Autodesk Inventor part; units mm, degrees
ref_plane "YZ Plane" through (0, 0, 0) normal (1, 0, 0) x (0, 1, 0)
ref_plane "XZ Plane" through (0, 0, 0) normal (0, 1, 0) x (-1, 0, 0)
ref_plane "XY Plane" through (0, 0, 0) normal (0, 0, 1) x (1, 0, 0)
sketch "Sketch1" plane through (0, 0, 0) normal (0, 0, 1) x (1, 0, 0)
  line L0 (-85, 50) -> (85, 50)
  line L1 (85, 50) -> (85, -50)
  line L2 (85, -50) -> (-85, -50)
  line L3 (-85, -50) -> (-85, 50)
  line L4 (-85, 50) -> (85, -50) construction
  line L5 (85, 50) -> (-85, -50) construction
  point P0 (0, 0)
  dimension "d0" = 170
  dimension "d1" = 100
extrude "Extrusion1" add sketch "Sketch1" along normal mid plane 10
sketch "Sketch2" plane through (0, 0, 5) normal (0, 0, 1) x (1, 0, 0)
  line L0 (-85, 50) -> (-85, -50)
  line L1 (-85, -50) -> (85, -50)
  line L2 (85, -50) -> (85, 50)
  line L3 (85, 50) -> (-85, 50)
  point P0 (0, 0)
  point P1 (-80, -45)
  point P2 (0, -45)
  point P3 (-55, -45)
  point P4 (55, -45)
  point P5 (0, -45)
  point P6 (80, -45)
  point P7 (-80, 0)
  point P8 (80, 0)
  point P9 (-80, 45)
  point P10 (80, 45)
  point P11 (-55, 45)
  point P12 (0, 45)
  point P13 (55, 45)
  dimension "d4" = 5
  dimension "d5" = 5
  dimension "d8" = 80
  dimension "d13" = 25
  dimension "d14" = 5
  dimension "d16" = 5
  dimension "d60" = 5
  dimension "d61" = 5
  dimension "d62" = 25
  dimension "d65" = 45
  dimension "d72" = 90
hole "Hole1" at (-80, -45, 5) at (0, -45, 5) at (-55, -45, 5) at (55, -45, 5) at (-80, 45, 5) at (-80, 0, 5) at (-55, 45, 5) at (0, 45, 5) at (55, 45, 5) at (80, 45, 5) at (80, 0, 5) at (80, -45, 5) direction (0, 0, -1) diameter 3.242 end through all
sketch "Sketch3" plane through (0, 0, 5) normal (0, 0, 1) x (1, 0, 0)
  point P0 (0, 0)
  point P1 (0, 15)
  point P2 (-15, 0)
  point P3 (0, -15)
  point P4 (15, 0)
  dimension "d105" = 15
  dimension "d108" = 360
hole "Hole2" at (0, 15, 5) at (-15, 0, 5) at (0, -15, 5) at (15, 0, 5) direction (0, 0, -1) diameter 3 depth 5 tip angle 118
properties part number "topwindow"
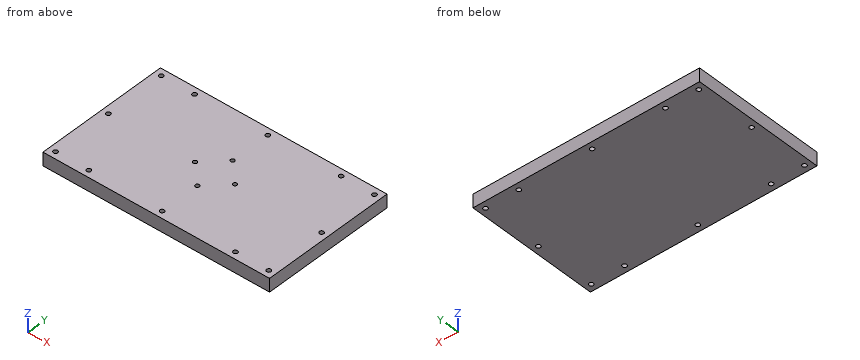
Geometry check sheet. Reference: the model listing, model coordinates, mm. Round coordinates to 2 decimals unless told otherwise and drop trailing zeros. Write each loop counter-clockwise with the first axis right and the second up, starting at its lowest first coordinate (ties: lowest second). Pieces come first, ordered by that corner, then holes. Notation, with made-up numbers: (43, 21) -> (61, 21) arc R13 cw to (61, 39) -> close; hole circle Ø4 at (13, 7.25). An arc over 180 degrees is marked (long way). One line per item, written item: value. Start each with the question number.
(1) Scan lines: line 1 (Y direction, x = 0, z = 2.9); line 2 (X direction, y = 45, z = 0.5); line 3 (X direction, y = 0, z = 3.55). Record each from-to range of solid material in increasing order. Write a range as [from, to].
(2) Cross-section at A-A, the plane x = 80. Record the cut outline in (y, z), and give its area (3 significant figures).
(3) Cross-section at B-B, the plane x = 55. Record the cut outline in (y, z), and give its area (3 significant figures).
(4) Go/stop test with flat-tipped pins: pin 1 Ø1.8 at (x, y) = (0, 15) entering from +Z; pin 2 Ø2.5 at (x, y) = (-15, 0) entering from +Z. Record where each tip stops, or that it passes through.
Answer:
1. line 1: [-50, -46.62], [-43.38, -16.5], [-13.5, 13.5], [16.5, 43.38], [46.62, 50]
1. line 2: [-85, -81.62], [-78.38, -56.62], [-53.38, -1.62], [1.62, 53.38], [56.62, 78.38], [81.62, 85]
1. line 3: [-85, -81.62], [-78.38, -16.5], [-13.5, 13.5], [16.5, 78.38], [81.62, 85]
2. outline: (-50, -5) -> (-46.62, -5) -> (-46.62, 5) -> (-50, 5) -> close; (-43.38, -5) -> (-1.62, -5) -> (-1.62, 5) -> (-43.38, 5) -> close; (1.62, -5) -> (43.38, -5) -> (43.38, 5) -> (1.62, 5) -> close; (46.62, -5) -> (50, -5) -> (50, 5) -> (46.62, 5) -> close
2. area: 903 mm²
3. outline: (-50, -5) -> (-46.62, -5) -> (-46.62, 5) -> (-50, 5) -> close; (-43.38, -5) -> (43.38, -5) -> (43.38, 5) -> (-43.38, 5) -> close; (46.62, -5) -> (50, -5) -> (50, 5) -> (46.62, 5) -> close
3. area: 935 mm²
4. pin 1: z = -0.36
4. pin 2: z = -0.15
